Autodesk Inventor part; units mm, degrees
ref_plane "Work Plane1" through (29.85, 0, 0) normal (1, 0, 0) x (0, 1, 0)
ref_plane "XZ Plane" through (0, 0, 0) normal (0, 1, 0) x (-1, 0, 0)
ref_plane "XY Plane" through (0, 0, 0) normal (0, 0, 1) x (1, 0, 0)
sketch "Sketch1" plane through (0, 0, 0) normal (0, 0, 1) x (1, 0, 0)
  circle A0 centre (0, 0) radius 35
  dimension "d0" = 70
extrude "Extrusion1" add sketch "Sketch1" along normal blind 6
sketch "Sketch2" plane through (0, 0, 6) normal (0, 0, 1) x (1, 0, 0)
  circle A0 centre (0, 0) radius 35
  circle A1 centre (0, 0) radius 30
  dimension "d3" = 60
extrude "Extrusion2" cut sketch "Sketch2" against normal blind 3 contours A1
sketch "Sketch3" plane through (0, 0, 0) normal (0, 0, -1) x (-1, 0, 0)
  circle A0 centre (0, 0) radius 35
  circle A1 centre (0, 0) radius 29.35
  circle A2 centre (0, 0) radius 27.85
  dimension "d6" = 58.7
  dimension "d7" = 55.7
extrude "Extrusion3" add sketch "Sketch3" along normal blind 25 contours A1
fillet "Fillet1" radius 2 1 edges at (-35, 0, 6)
sketch "Sketch4" plane through (0, 0, 3) normal (0, 0, 1) x (1, 0, 0)
  circle A0 centre (0, 0) radius 30
  circle A1 centre (0, 0) radius 12.5
  dimension "d11" = 25
extrude "Extrusion4" cut sketch "Sketch4" against normal blind 10 contours A1
ref_plane "Work Plane1" through (29.85, 0, 0) normal (1, 0, 0) x (0, 1, 0)
sketch "Sketch5" plane through (29.85, 0, 0) normal (1, 0, 0) x (0, 1, 0)
  line L0 (-10, -17) -> (10, -17)
  line L1 (10, -17) -> (10, -28.5985)
  line L2 (10, -28.5985) -> (-10, -28.5985)
  line L3 (-10, -28.5985) -> (-10, -17)
  line L4 (0, -31.2) -> (0, 12.2)
  line L5 (0, 0) -> (-49, 0)
  dimension "d15" = 20
  dimension "d17" = 17
extrude "Extrusion5" cut sketch "Sketch5" against normal blind 10
properties part number "Tapa_superior_carcasa"
The listing builds one solid part. Answer for the finished solid, in the listing's coordinates (mm). A direction names the side the tool comes from. Coordinates: 2 decimals unless noted, no trailing zeros. Order: outer loops, then holes, each group sorted by start corner. A loop starts at its lowest first (then second) coordinate and runs counter-clockwise, first axis right, second up.
Q1. A cutting plane is placed at D-D, the plane z = -19. Write down the section's boundary in (x, y).
Q2. A cutting plane is placed at A-A, the plane x = 0. Write down the section's boundary in (y, z), and give its area (3 significant figures).
Q3. Which of the six approach directions +Z, -Z, +X, -X, +Y, -Y give full straight-line access (tool end or side, diameter ignored) to faces 1 (the face through (28.1, -0.1, -17)), 2 (the face through (-28, -8.8, -12.3)), 3 (the face through (-29.97, 1.32, 4.52))?
Q4. Consider line 1 (Y direction, x = 0, z = -19.5); line 2 (X direction, y = -1, z = -14.5); line 3 (Z direction, x = -14, y = 7). Determine where each line is inside the solid, lowest interval first.
Q5. A cutting plane is placed at B-B, the plane y = 0. Write down the section's boundary in (x, z).
Q6. For a pull along Y with two mould halves and no side action, classify faces 4 (the face through (-28, 21, 2)), 5 (the face through (27, -10, -21)), 6 (the face through (-28.2, 0.1, -25)) as pulls with the +Y half, pulls with the -Y half, needs draft (parallel to the pull), parting line crosses it, or undercut.
Q7. A cutting plane is placed at C-C, the plane z = -2.5. Write down the section's boundary in (x, y), and give its area (3 significant figures).
Q8. Given P1, Ø8, axis at x = 6.5, y = 2.5, coming from the +Z side; P2, Ø0.5, axis at x = 26.5, z = -23, coming from the -Y side; P3, Ø6, axis at x = 21.5, z = -16, coming from the +Y side; P4, Ø3, axis at y = 5.5, z = -12, coming from the -X side, each flat-ended and moving along its own axis, determine where each tip first touches the part or whether it passes through.
Answers follow:
1. outline: (25.99, -10) arc R27.85 cw (long way) to (25.99, 10) - (27.59, 10) arc R29.35 ccw (long way) to (27.59, -10) - close
2. outline: (-35, 0) - (-29.35, 0) - (-29.35, -25) - (-27.85, -25) - (-27.85, 0) - (-12.5, 0) - (-12.5, 3) - (-30, 3) - (-30, 6) - (-33, 6) arc R2 ccw to (-35, 4) - close; (12.5, 0) - (27.85, 0) - (27.85, -25) - (29.35, -25) - (29.35, 0) - (35, 0) - (35, 4) arc R2 ccw to (33, 6) - (30, 6) - (30, 3) - (12.5, 3) - close
2. area: 238 mm2
3. face 1: -Z, +X
3. face 2: -Z
3. face 3: +Z
4. line 1: y = -29.35 to -27.85, 27.85 to 29.35
4. line 2: x = -29.33 to -27.83, 27.83 to 29.33
4. line 3: z = 0 to 3
5. outline: (-35, 0) - (-29.35, 0) - (-29.35, -25) - (-27.85, -25) - (-27.85, 0) - (-12.5, 0) - (-12.5, 3) - (-30, 3) - (-30, 6) - (-33, 6) arc R2 ccw to (-35, 4) - close; (12.5, 0) - (27.85, 0) - (27.85, -17) - (29.35, -17) - (29.35, 0) - (35, 0) - (35, 4) arc R2 ccw to (33, 6) - (30, 6) - (30, 3) - (12.5, 3) - close
6. face 4: parting line crosses it
6. face 5: undercut
6. face 6: needs draft
7. outline: circle Ø58.7 at (0, 0); hole circle Ø55.7 at (0, 0)
7. area: 270 mm2
8. P1: passes through
8. P2: stops at y = -13.13
8. P3: stops at y = 22.79
8. P4: stops at x = -29.08
